Geometry check sheet. Reference: the model listing, model coordinates, mm. Face numbers are marked on the shaded views. A direction names the side the tool comes from. Round coordinates to 2 decimals unless told otherwise and drop trailing zeros. Write each loop counter-clockwise with the first axis right and the second up, starting at its lowest first coordinate (ties: lowest second). Pieces come first, ordered by that corner, then holes. Notation, with made-up numbers: M 87.25,33.25 L 123.25,33.25 A28 ccw 123.25,62.25 Z; hole C -26.75,-31 d11. An arc over 180 degrees is marked long. Answer in a Markdown table with one row per item. Add a question column.
from build123d import *

# Parameters (mm, degrees)
PAD_DEPTH       = 180
SKETCH001_W     = 168
SKETCH001_H     = 210
POCKET_DEPTH    = 175
SKETCH002_W     = 210
SKETCH002_H     = 181.4
POCKET001_DEPTH = 175
POCKET002_DEPTH = 5.5
SKETCH004_W     = 10.5
SKETCH004_H     = 21.8
POCKET003_DEPTH = 5.5
SKETCH005_R     = 3.2
POCKET004_DEPTH = 100
SKETCH006_W     = 15.4
SKETCH006_H     = 20.4
POCKET005_DEPTH = 5
SKETCH007_R     = 20
POCKET006_DEPTH = 5
SKETCH008_R     = 19
SKETCH008_R_2   = 2.2
POCKET007_DEPTH = 180.001
SKETCH052_R     = 5.049841
POCKET042_DEPTH = 5


with BuildPart() as part:
    # Sketch → Pad (new body)
    with BuildSketch(Plane.XY):
        with BuildLine():
            Line((-100, 110), (100, 110))
            ThreePointArc((110, 100), (107.071068, 107.071068), (100, 110))
            Line((110, 100), (110, -100))
            ThreePointArc((100, -110), (107.071068, -107.071068), (110, -100))
            Line((100, -110), (-100, -110))
            ThreePointArc((-110, -100), (-107.071068, -107.071068), (-100, -110))
            Line((-110, -100), (-110, 100))
            ThreePointArc((-100, 110), (-107.071068, 107.071068), (-110, 100))
        make_face()
    extrude(amount=PAD_DEPTH)

    # Sketch001 (on DatumPlane) → Pocket (cut)
    with BuildSketch(Plane.XY.offset(180)):
        Rectangle(SKETCH001_W, SKETCH001_H)
    extrude(amount=-POCKET_DEPTH, mode=Mode.SUBTRACT)

    # Sketch002 (on DatumPlane) → Pocket001 (cut)
    with BuildSketch(Plane.XY.offset(180)):
        Rectangle(SKETCH002_W, SKETCH002_H)
    extrude(amount=-POCKET001_DEPTH, mode=Mode.SUBTRACT)

    # Sketch003 (on DatumPlane) → Pocket002 (cut)
    with BuildSketch(Plane.XY.offset(175)):
        Polygon((89.39045, 96.15), (94.5, 93.2), (99.60955, 96.15), (99.60955, 102.05), (94.5, 105), (89.39045, 102.05), align=None)
        Polygon((99.60955, -102.05), (99.60955, -96.15), (94.5, -93.2), (89.39045, -96.15), (89.39045, -102.05), (94.5, -105), align=None)
        Polygon((-89.39045, -102.05), (-89.39045, -96.15), (-94.5, -93.2), (-99.60955, -96.15), (-99.60955, -102.05), (-94.5, -105), align=None)
        Polygon((-89.39045, 96.15), (-89.39045, 102.05), (-94.5, 105), (-99.60955, 102.05), (-99.60955, 96.15), (-94.5, 93.2), align=None)
    extrude(amount=-POCKET002_DEPTH, mode=Mode.SUBTRACT)

    # Sketch004 (on DatumPlane) → Pocket003 (cut)
    with BuildSketch(Plane.XY.offset(175)):
        with Locations((-94.5, 88.2)):
            Rectangle(SKETCH004_W, SKETCH004_H)
        with Locations((94.5, 88.2)):
            Rectangle(SKETCH004_W, SKETCH004_H)
        with Locations((-94.5, -88.2)):
            Rectangle(SKETCH004_W, SKETCH004_H)
        with Locations((94.5, -88.2)):
            Rectangle(SKETCH004_W, SKETCH004_H)
    extrude(amount=-POCKET003_DEPTH, mode=Mode.SUBTRACT)

    # Sketch005 (on DatumPlane) → Pocket004 (cut)
    with BuildSketch(Plane.XY.offset(180)):
        with Locations((-94.5, 99.1)):
            Circle(SKETCH005_R)
        with Locations((94.5, 99.1)):
            Circle(SKETCH005_R)
        with Locations((-94.5, -99.1)):
            Circle(SKETCH005_R)
        with Locations((94.5, -99.1)):
            Circle(SKETCH005_R)
    extrude(amount=-POCKET004_DEPTH, mode=Mode.SUBTRACT)

    # Sketch006 (on DatumPlane) → Pocket005 (cut)
    with BuildSketch(Plane.YZ.offset(110)):
        with Locations((-47.5, 97.7)):
            Rectangle(SKETCH006_W, SKETCH006_H)
    extrude(amount=-POCKET005_DEPTH, mode=Mode.SUBTRACT)

    # Sketch007 (on DatumPlane) → Pocket006 (cut)
    with BuildSketch(Plane.XZ.offset(-110)):
        with Locations((0, 125)):
            Circle(SKETCH007_R)
    extrude(amount=POCKET006_DEPTH, mode=Mode.SUBTRACT)

    # Sketch008 (on DatumPlane) → Pocket007 (cut, through all)
    with BuildSketch(Plane.XY.offset(180)):
        with Locations((0, -7)):
            Circle(SKETCH008_R)
        with Locations((0, 28)):
            Circle(SKETCH008_R_2)
        with Locations((28, 0)):
            Circle(SKETCH008_R_2)
        with Locations((-28, 0)):
            Circle(SKETCH008_R_2)
        with Locations((0, -33)):
            Circle(SKETCH008_R_2)
    extrude(amount=-POCKET007_DEPTH, mode=Mode.SUBTRACT)

    # Sketch052 (on Face37 of Pocket007) → Pocket042 (cut)
    with BuildSketch(Plane.XY.offset(5)):
        with Locations((0, -67.5)):
            Circle(SKETCH052_R)
    extrude(amount=-POCKET042_DEPTH, mode=Mode.SUBTRACT)


solid = part.part
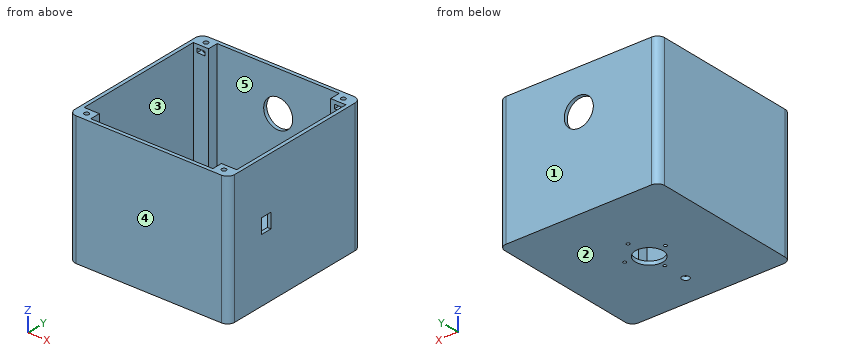
Item 1: Section check A-A, the plane y = -7. Record the boundary of the cut face in (x, z), and give its area (3 significant figures).
Item 2: Access from +Z, -Z, +X, -X, +Y, -Y to the whole of each face (thin tool, end or side, straight path). Record for the marked faces 4 and 5.
Item 3: Mould release check, pull along Y, two halves, no side actions. Record for the marked faces 1, 2 and 3: +Y half, -Y half, draft (parallel to the pull), parting line (faces both ways), or undercut.
Item 4: Section check D-D, the plane y = 39. Record the boundary of the cut face in (x, z), and give its area (3 significant figures).
Item 5: Section check C-C, the plane z = 125. Record the boundary of the cut face in (x, y).
Item 6: Gauge pin test, flat ends, axial feed: pin 1 Ø8 at (x, y) = (88, 10) entering from +Z; pin 2 Ø2.5 at (x, z) = (106.5, 96) entering from -Y. Record the tip position at first contact, or that the pin passes through.
Item 7: Scan lines: probe 1 along Y at (x, z) = (94.5, 125); probe 2 along Y at (x, z) = (0, 1); probe 3 along X at (y, z) = (-99, 101). Record each from-to range of solid material in increasing order. Write a range as from..to.
Item 8: Section check B-B, the plane z = 58. Record the boundary of the cut face in (x, y), and give its area (3 significant figures).
Result sheet:
| question | item | result |
|---|---|---|
| 1 | outline | M -110,0 L -19,0 L -19,5 L -105,5 L -105,180 L -110,180 Z; M 19,0 L 110,0 L 110,180 L 105,180 L 105,5 L 19,5 Z |
| 1 | area | 2,660 mm^2 |
| 2 | face 4 | +Z, -Z, +X, -X, -Y |
| 2 | face 5 | +Z |
| 3 | face 1 | +Y half |
| 3 | face 2 | draft |
| 3 | face 3 | undercut |
| 4 | outline | M -110,0 L 110,0 L 110,180 L 105,180 L 105,5 L -105,5 L -105,180 L -110,180 Z |
| 4 | area | 2,850 mm^2 |
| 5 | outline | M -110,-100 A10 ccw -100,-110 L 100,-110 A10 ccw 110,-100 L 110,100 A10 ccw 100,110 L 20,110 L 20,105 L 84,105 L 84,90.7 L 105,90.7 L 105,-90.7 L 84,-90.7 L 84,-105 L -84,-105 L -84,-90.7 L -105,-90.7 L -105,90.7 L -84,90.7 L -84,105 L -20,105 L -20,110 L -100,110 A10 ccw -110,100 Z; hole C -94.5,-99.1 d6.4; hole C -94.5,99.1 d6.4; hole C 94.5,-99.1 d6.4; hole C 94.5,99.1 d6.4 |
| 6 | pin 1 | stops at z = 5 |
| 6 | pin 2 | stops at y = -108.51 |
| 7 | probe 1 | y = -110..-102.3, -95.9..-90.7, 90.7..95.9, 102.3..110 |
| 7 | probe 2 | y = -110..-72.55, -62.45..-35.2, -30.8..-26, 12..25.8, 30.2..110 |
| 7 | probe 3 | x = -110..-97.7, -91.3..-84, 84..91.3, 97.7..110 |
| 8 | outline | M -110,-100 A10 ccw -100,-110 L 100,-110 A10 ccw 110,-100 L 110,100 A10 ccw 100,110 L -100,110 A10 ccw -110,100 Z; hole M -105,-90.7 L -84,-90.7 L -84,-105 L 84,-105 L 84,-90.7 L 105,-90.7 L 105,90.7 L 84,90.7 L 84,105 L -84,105 L -84,90.7 L -105,90.7 Z |
| 8 | area | 5,420 mm^2 |
